Can you work these out from the model? Positions are in its coordinate system, mm. A direction names the side the tool comes from. Round coordinates to 2 decimals unless told otherwise and drop trailing zeros. Order: outer loops, then holes, each group sorted by start corner. A loop starts at its lowest first (then second) coordinate and runs counter-clockwise, first axis right, second up. Notation, with made-up numbers: (45, 30.25) -> (54, 30.25) arc R13 cw to (54, 45.25) -> close; hole circle Ø11 at (20.5, 53). An arc over 180 degrees is marked (long way). Use a Markdown table: item, result. Add a question column.
Q1. I'm going to push flat-ended pins straight in: pin 1 Ø2 at (x, z) = (-11, 12) entering from -Y; pin 2 Ø1 at (y, z) = (-13, -8.5) entering from +X; pin 3 Ø8 at (x, y) = (-12.5, 10.5) entering from -Z. Where does each tip first touch, or does it pass through?
Q2. We'd pull the mould along X, two halves only. Please class faces 4 (the face through (-21.2, -43, 0.1)), 5 (the face through (-23.977, -3.806, 1.055)), 6 (the face through (0, 42, 10)): +X half, -X half, draft (parallel to the pull), parting line (faces both ways), or undercut.
Q3. I need wall thicknesses on line 1 along Z through (x, y) = (0, -33); line 2 along Y through (x, z) = (14.5, -10); line 3 along Y through (x, z) = (6.5, -11). Which ranges of each line are inside material? Lowest first, please. Write a range as [from, to].
Q4. If we section it at B-B on y = -24.5: List the corners of the cut face in (x, z) for me, plus the area to 3 significant figures.
Q5. If we section it at A-A on x = 0: List the corners of the cut face in (y, z) for me.
Q6. For faces 1 (the face through (3.78, 42.2, 2.9)), 2 (the face through (0, 43, 0)), 3 (the face through (0, -30, 0)), which set-ups out of +Z, -Z, +X, -X, +Y, -Y let a thin tool reach every point of the face, with its end or its side?
Q7. If we section it at C-C on y = 38: List the corners of the cut face in (x, z) for me.
Solid Edge part; units mm, degrees
sketch "Sketch1" plane through (0, 0, 0) normal (0, -1, 0) x (1, 0, 0)
  circle A0 centre (0, 0) radius 24
extrude "Protrusion1" add sketch "Sketch1" along normal mid plane 86
fillet "Round1" radius 6.5 1 edges at (-24, 43, 0)
sketch "Sketch2" plane through (0, 43, 0) normal (0, 1, 0) x (-1, 0, 0)
  line L0 (-10, 0) -> (-10, -16)
  arc A0 (-10, 0) -> (10, 0) centre (0, 0) cw
  line L1 (10, 0) -> (10, -16)
extrude "Cutout1" cut sketch "Sketch2" against normal blind 1.5875 material side at (9.95, 43, -8)
sketch "Sketch3" plane through (0, 41.4125, -6.0688) normal (0, 1, 0) x (-1, 0, 0)
  circle A0 centre (0, 6.0688) radius 4.7625
extrude "Protrusion2" add sketch "Sketch3" along normal blind 1.5875
sketch "Sketch4" plane through (0, -43, 0) normal (0, -1, 0) x (1, 0, 0)
  circle A0 centre (0, 0) radius 21
extrude "Cutout2" cut sketch "Sketch4" against normal blind 13
properties part number "COIL-X1A" material "PURCHASED"
Answer below:
| question | item | result |
|---|---|---|
| 1 | pin 1 | y = -30 |
| 1 | pin 2 | x = 22.63 |
| 1 | pin 3 | z = -22.44 |
| 2 | face 4 | draft |
| 2 | face 5 | parting line |
| 2 | face 6 | undercut |
| 3 | line 1 | [-24, -21], [21, 24] |
| 3 | line 2 | [-30, 43] |
| 3 | line 3 | [-30, 41.41] |
| 4 | outline | circle Ø48 at (0, 0) |
| 4 | area | 1,810 mm² |
| 5 | outline | (-43, -24) -> (36.5, -24) arc R6.5 ccw to (41.41, -21.76) -> (41.41, -4.76) -> (43, -4.76) -> (43, 4.76) -> (41.41, 4.76) -> (41.41, 10) -> (43, 10) -> (43, 17.5) arc R6.5 ccw to (36.5, 24) -> (-43, 24) -> (-43, 21) -> (-30, 21) -> (-30, -21) -> (-43, -21) -> close |
| 6 | face 1 | +Y |
| 6 | face 2 | +Z, -Z, +X, -X, +Y |
| 6 | face 3 | -Y |
| 7 | outline | circle Ø47.65 at (0, 0) |
